from build123d import *
from OCP.BRepFilletAPI import BRepFilletAPI_MakeChamfer

# Parameters (mm, degrees)
SKETCH1_W                       = 16.6
SKETCH1_H                       = 11.5
BOSS_EXTRUDE1_DEPTH             = 10
SKETCH2_W                       = 21
SKETCH2_H                       = 14.8
BOSS_EXTRUDE2_DEPTH             = 1.5
SKETCH3_W                       = 0.5
SKETCH3_H                       = 5
BOSS_EXTRUDE3_DEPTH             = 8
SKETCH4_W                       = 0.5
SKETCH4_H                       = 0.4
CUT_EXTRUDE1_DEPTH              = 22.623424798
BOSS_EXTRUDE4_REACH             = 19.241
SKETCH5_W                       = 0.75
SKETCH5_H                       = 2.5
BOSS_EXTRUDE4_DIRECTION_2_REACH = 19.241
BOSS_EXTRUDE5_DEPTH             = 2.8
CHAMFER1_SIZE                   = 1.8
CHAMFER1_SIZE_2                 = 1.039230485
BOSS_EXTRUDE6_DEPTH             = 4.65
SKETCH8_W                       = 1.1
SKETCH8_H                       = 0.45
BOSS_EXTRUDE7_DEPTH             = 1.9
CHAMFER2_SIZE                   = 0.5
CHAMFER2_SIZE2                  = 0.288675135


with BuildPart() as part:
    # Sketch1 → Boss-Extrude1 (new body)
    with BuildSketch(Plane.XY):
        Rectangle(SKETCH1_W, SKETCH1_H)
    extrude(amount=BOSS_EXTRUDE1_DEPTH)

    # Sketch2 → Boss-Extrude2 (add)
    with BuildSketch(Plane.XY.offset(10)):
        Rectangle(SKETCH2_W, SKETCH2_H)
    extrude(amount=BOSS_EXTRUDE2_DEPTH)

    # Sketch3 → Boss-Extrude3 (add)
    with BuildSketch(Plane(origin=(0, 0, 0), x_dir=(-1, 0, 0), z_dir=(0, 0, -1))):
        Rectangle(SKETCH3_W, SKETCH3_H)
        with Locations((-6, 0)):
            Rectangle(SKETCH3_W, SKETCH3_H)
    extrude(amount=BOSS_EXTRUDE3_DEPTH)

    # Sketch4 → Cut-Extrude1 (cut, through all)
    with BuildSketch(Plane(origin=(6.25, 0, 0), x_dir=(0, 0, -1), z_dir=(1, 0, 0))):
        Polygon((6.5, 2.5), (8, 1.449688693), (8, 2.5), align=None)
        Polygon((8, -2.5), (8, -1.449688693), (6.5, -2.5), align=None)
        with Locations((2.25, -2.3)):
            Rectangle(SKETCH4_W, SKETCH4_H)
        with BuildLine():
            ThreePointArc((0, -0.75), (0.530330086, -0.530330086), (0.75, 0))
            Line((0.75, 0), (0, 0))
            Line((0, 0), (0, -0.75))
        make_face()
        with BuildLine():
            Line((0, 0), (0.75, 0))
            ThreePointArc((0.75, 0), (0.530330086, 0.530330086), (0, 0.75))
            Line((0, 0.75), (0, 0))
        make_face()
        with Locations((2.25, 2.3)):
            Rectangle(SKETCH4_W, SKETCH4_H)
        with BuildLine():
            Line((4.25, 0), (6.3, 0))
            Line((6.3, 0), (5.432692308, 0.612598863))
            ThreePointArc((5.432692308, 0.612598863), (4.655050171, 0.665965176), (4.25, 0))
        make_face()
        with BuildLine():
            Line((5.432692308, -0.612598863), (6.3, 0))
            Line((6.3, 0), (4.25, 0))
            ThreePointArc((4.25, 0), (4.655050171, -0.665965176), (5.432692308, -0.612598863))
        make_face()
    extrude(amount=-CUT_EXTRUDE1_DEPTH, mode=Mode.SUBTRACT)

    # Boss-Extrude4: up to this face of the body (flat: up to its plane)
    boss_extrude4_end = Plane(part.part.faces().sort_by_distance((0, 5.75, 5))[0])
    # Sketch5 → Boss-Extrude4 (add, up to the picked face)
    with BuildSketch(Plane(origin=(0, 0, 0), x_dir=(1, 0, 0), z_dir=(0, 1, 0)), mode=Mode.PRIVATE) as boss_extrude4_sk1:
        with Locations((-8.675, -1.25)):
            Rectangle(SKETCH5_W, SKETCH5_H)
    boss_extrude4_tool1 = split(extrude(boss_extrude4_sk1.sketch, amount=BOSS_EXTRUDE4_REACH, mode=Mode.PRIVATE), bisect_by=boss_extrude4_end, keep=Keep.BOTH, mode=Mode.PRIVATE)
    boss_extrude4 = boss_extrude4_tool1.solids().sort_by(Axis((-8.675, 0, 1.25), (0, 1, 0)))[0]
    add(boss_extrude4)

    # Boss-Extrude4 direction 2: up to this face of the body (flat: up to its plane)
    boss_extrude4_direction_2_end = Plane(part.part.faces().sort_by_distance((0, -5.75, 5))[0])
    # Sketch5 → Boss-Extrude4 direction 2 (add, up to the picked face)
    with BuildSketch(Plane(origin=(0, 0, 0), x_dir=(1, 0, 0), z_dir=(0, 1, 0)), mode=Mode.PRIVATE) as boss_extrude4_direction_2_sk1:
        with Locations((-8.675, -1.25)):
            Rectangle(SKETCH5_W, SKETCH5_H)
    boss_extrude4_direction_2_tool1 = split(extrude(boss_extrude4_direction_2_sk1.sketch, amount=-BOSS_EXTRUDE4_DIRECTION_2_REACH, mode=Mode.PRIVATE), bisect_by=boss_extrude4_direction_2_end, keep=Keep.BOTH, mode=Mode.PRIVATE)
    boss_extrude4_direction_2 = boss_extrude4_direction_2_tool1.solids().sort_by(Axis((-8.675, 0, 1.25), (0, -1, 0)))[0]
    add(boss_extrude4_direction_2)

    # Mirror1: Boss-Extrude4, Boss-Extrude4 direction 2 across plane
    add(boss_extrude4.mirror(Plane(origin=(0, 0, 0), x_dir=(0, 0, 1), z_dir=(1, 0, 0))))
    add(boss_extrude4_direction_2.mirror(Plane(origin=(0, 0, 0), x_dir=(0, 0, 1), z_dir=(1, 0, 0))))

    # Sketch6 → Boss-Extrude5 (add, symmetric)
    with BuildSketch(Plane(origin=(0, 0, 0), x_dir=(1, 0, 0), z_dir=(0, 1, 0))):
        with BuildLine():
            Line((-8.3, -2.5), (-9.05, -2.5))
            Line((-9.05, -2.5), (-10.056775734, -6.054415838))
            ThreePointArc((-10.056775734, -6.054415838), (-10.16130334, -6.692525863), (-10.056775734, -7.330635888))
            Line((-10.056775734, -7.330635888), (-9.03, -10))
            Line((-9.03, -10), (-8.3, -10))
            Line((-8.3, -10), (-8.3, -9.83))
            Line((-8.3, -9.83), (-9.324133061, -7.167955242))
            ThreePointArc((-9.324133061, -7.167955242), (-9.430562185, -6.777402526), (-9.37345004, -6.376657238))
            Line((-9.37345004, -6.376657238), (-8.3, -2.62))
            Line((-8.3, -2.62), (-8.3, -2.5))
        make_face()
    boss_extrude5 = extrude(amount=BOSS_EXTRUDE5_DEPTH, both=True)

    # Mirror2: Boss-Extrude5 across plane
    add(boss_extrude5.mirror(Plane(origin=(0, 0, 0), x_dir=(0, 0, 1), z_dir=(1, 0, 0))))

    # Chamfer1
    # the kernel refuses this chamfer: 1.8, 1.039230485 mm, written as the material it takes off along each edge
    with BuildSketch(Plane(origin=(-15.156754358, 7.4, 11.5), x_dir=(0, 0.019326765612700948, -0.9998132206222079), z_dir=(1, 0, 0))) as chamfer1_piece_1:
        Polygon((CHAMFER1_SIZE * 0.999813220622, -CHAMFER1_SIZE * 0.0193267656127), (-CHAMFER1_SIZE_2 * 0.0193267656042, -CHAMFER1_SIZE_2 * 0.999813220181), (0, 0), align=None)
    extrude(amount=30.313508717, mode=Mode.SUBTRACT)
    with BuildSketch(Plane(origin=(-10.5, -12.056754358, 11.5), x_dir=(-0.019326765612700473, 0, -0.9998132206222079), z_dir=(0, 1, 0)), Plane(origin=(10.5, 12.056754358, 11.5), x_dir=(0.019326765612700473, 0, -0.9998132206222079), z_dir=(0, -1, 0))) as chamfer1_piece_2:
        Polygon((CHAMFER1_SIZE * 0.999813220622, -CHAMFER1_SIZE * 0.0193267656127), (-CHAMFER1_SIZE_2 * 0.0193267656042, -CHAMFER1_SIZE_2 * 0.999813220181), (0, 0), align=None)
    extrude(amount=24.113508717, mode=Mode.SUBTRACT)
    with BuildSketch(Plane(origin=(15.156754358, -7.4, 11.5), x_dir=(0, 0.9983227437537925, 0.05789386240267112), z_dir=(-1, 0, 0))) as chamfer1_piece_3:
        Polygon((CHAMFER1_SIZE_2 * 0.998322743313, CHAMFER1_SIZE_2 * 0.0578938623771), (-CHAMFER1_SIZE * 0.0578938624027, CHAMFER1_SIZE * 0.998322743754), (0, 0), align=None)
    extrude(amount=30.313508717, mode=Mode.SUBTRACT)

    # Sketch7 → Boss-Extrude6 (add, symmetric)
    with BuildSketch(Plane(origin=(0, 0, 0), x_dir=(1, 0, 0), z_dir=(0, 1, 0))):
        with BuildLine():
            Line((-7.960769515, -11.5), (7.960769515, -11.5))
            ThreePointArc((7.960769515, -11.5), (1.177888648, -13.404715365), (-4.995235012, -16.8))
            Line((-4.995235012, -16.8), (-7.960769515, -11.5))
        make_face()
    extrude(amount=BOSS_EXTRUDE6_DEPTH, both=True)

    # Sketch8 → Boss-Extrude7 (add)
    with BuildSketch(Plane(origin=(0, 0, 10), x_dir=(-1, 0, 0), z_dir=(0, 0, -1))):
        with Locations((-2.48, 5.975)):
            Rectangle(SKETCH8_W, SKETCH8_H)
        with Locations((-2.48, -5.975)):
            Rectangle(SKETCH8_W, SKETCH8_H)
        with Locations((-7.43, 5.975)):
            Rectangle(SKETCH8_W, SKETCH8_H)
        with Locations((-7.43, -5.975)):
            Rectangle(SKETCH8_W, SKETCH8_H)
        with Locations((2.48, -5.975)):
            Rectangle(SKETCH8_W, SKETCH8_H)
        with Locations((7.43, -5.975)):
            Rectangle(SKETCH8_W, SKETCH8_H)
        with Locations((2.48, 5.975)):
            Rectangle(SKETCH8_W, SKETCH8_H)
        with Locations((7.43, 5.975)):
            Rectangle(SKETCH8_W, SKETCH8_H)
    extrude(amount=BOSS_EXTRUDE7_DEPTH)

    # Chamfer2: one chamfer whose edges measure the first distance from different faces: ONE call of the kernel's chamfer builder (chamfer() names one face for all edges)
    chamfer2_edges_1 = [part.edges().sort_by_distance(p)[0] for p in [
        (2.48, 6.2, 8.1),
    ]]
    chamfer2_side_1 = [part.faces().sort_by_distance(p)[0] for p in [
        (2.48, 6.2, 9.05),
    ]]
    chamfer2_edges_2 = [part.edges().sort_by_distance(p)[0] for p in [
        (7.43, 6.2, 8.1),
    ]]
    chamfer2_side_2 = [part.faces().sort_by_distance(p)[0] for p in [
        (7.43, 6.2, 9.05),
    ]]
    chamfer2_edges_3 = [part.edges().sort_by_distance(p)[0] for p in [
        (2.48, -6.2, 8.1),
    ]]
    chamfer2_side_3 = [part.faces().sort_by_distance(p)[0] for p in [
        (2.48, -6.2, 9.05),
    ]]
    chamfer2_edges_4 = [part.edges().sort_by_distance(p)[0] for p in [
        (7.43, -6.2, 8.1),
    ]]
    chamfer2_side_4 = [part.faces().sort_by_distance(p)[0] for p in [
        (7.43, -6.2, 9.05),
    ]]
    chamfer2_edges_5 = [part.edges().sort_by_distance(p)[0] for p in [
        (-2.48, -6.2, 8.1),
    ]]
    chamfer2_side_5 = [part.faces().sort_by_distance(p)[0] for p in [
        (-2.48, -6.2, 9.05),
    ]]
    chamfer2_edges_6 = [part.edges().sort_by_distance(p)[0] for p in [
        (-7.43, -6.2, 8.1),
    ]]
    chamfer2_side_6 = [part.faces().sort_by_distance(p)[0] for p in [
        (-7.43, -6.2, 9.05),
    ]]
    chamfer2_edges_7 = [part.edges().sort_by_distance(p)[0] for p in [
        (-2.48, 6.2, 8.1),
    ]]
    chamfer2_side_7 = [part.faces().sort_by_distance(p)[0] for p in [
        (-2.48, 6.2, 9.05),
    ]]
    chamfer2_edges_8 = [part.edges().sort_by_distance(p)[0] for p in [
        (-7.43, 6.2, 8.1),
    ]]
    chamfer2_side_8 = [part.faces().sort_by_distance(p)[0] for p in [
        (-7.43, 6.2, 9.05),
    ]]
    chamfer2 = BRepFilletAPI_MakeChamfer(part.part.solid().wrapped)
    for e in chamfer2_edges_1:
        chamfer2.Add(CHAMFER2_SIZE, CHAMFER2_SIZE2, e.wrapped, chamfer2_side_1[0].wrapped)  # the first distance lies on this face
    for e in chamfer2_edges_2:
        chamfer2.Add(CHAMFER2_SIZE, CHAMFER2_SIZE2, e.wrapped, chamfer2_side_2[0].wrapped)  # the first distance lies on this face
    for e in chamfer2_edges_3:
        chamfer2.Add(CHAMFER2_SIZE, CHAMFER2_SIZE2, e.wrapped, chamfer2_side_3[0].wrapped)  # the first distance lies on this face
    for e in chamfer2_edges_4:
        chamfer2.Add(CHAMFER2_SIZE, CHAMFER2_SIZE2, e.wrapped, chamfer2_side_4[0].wrapped)  # the first distance lies on this face
    for e in chamfer2_edges_5:
        chamfer2.Add(CHAMFER2_SIZE, CHAMFER2_SIZE2, e.wrapped, chamfer2_side_5[0].wrapped)  # the first distance lies on this face
    for e in chamfer2_edges_6:
        chamfer2.Add(CHAMFER2_SIZE, CHAMFER2_SIZE2, e.wrapped, chamfer2_side_6[0].wrapped)  # the first distance lies on this face
    for e in chamfer2_edges_7:
        chamfer2.Add(CHAMFER2_SIZE, CHAMFER2_SIZE2, e.wrapped, chamfer2_side_7[0].wrapped)  # the first distance lies on this face
    for e in chamfer2_edges_8:
        chamfer2.Add(CHAMFER2_SIZE, CHAMFER2_SIZE2, e.wrapped, chamfer2_side_8[0].wrapped)  # the first distance lies on this face
    add(Compound.cast(chamfer2.Shape()), mode=Mode.REPLACE)


solid = part.part
The listing builds one solid part. Answer for the finished solid, in the listing's coordinates (mm). A direction names the side the tool comes from. Coordinates: 2 decimals unless noted, no trailing zeros. Loops run counter-clockwise (first coordinate to the right, second up) from the corner with the lowest first, then second, coordinate; pieces in that order, holes last. Notation, with made-up numbers: (60.5, 3) -> (97.5, 3) arc R22 ccw to (97.5, 28) -> close; hole circle Ø11 at (-18, -34). An arc over 180 degrees is marked (long way). Answer in a Markdown table with one row per item. Add a question column.
1. The part is cut by section B-B, the plane x = -1. Write down the section's boundary in (y, z).
2. Flat-ended cylindrical pins translate along their axes: P1, Ø0.6, axis at x = 2.5, z = 9, coming from the -Y side; P2, Ø4, axis at x = 6.5, z = 1, coming from the +Y side; P3, Ø5, axis at x = 8, z = -3.5, coming from the +Y side. Find the tip coordinate at first contact, or state that the pin passes through.
3. The part is cut by section A-A, the plane y = -4. Write down the section's boundary in (x, z), then the cut area to 3 significant figures.
4. The part is cut by section C-C, the plane y = 1.75. Count the separate pieces of the cut face and the enclosed holes in it, then the cut area to 3 significant figures.
5. Consider line 1 (Z direction, x = -8.75, y = -4.5); line 2 (X direction, y = -1.75, z = -1); line 3 (Z direction, x = -8, y = -3.75). Determine where each line is inside the solid, lowest interval first. Write a range as [from, to].
6. For faces 1 (the flat face through (-9.5, -2.8, 6.2)), 2 (the flat face through (-9.55, 0.04, 8.65)), 3 (the flat face through (9.05, 0, 1)), 4 (the flat face through (-2.5, 6.2, 9.3)), 5 (the flat face through (7.4, -6.2, 9.3)), determine the directions among +Z, -Z, +X, -X, +Y, -Y from which every point of the face is accessible in a straight line to the end or side of a thin tool.
7. Determine the mould class of faces 6 (the flat face through (-8.844, 0.039, 4.525)), 7 (the flat face through (0, 1.98, -7.24)), 8 (the cylindrical face through (1.269, 0.065, 13.367)) for opening direction X: +X half, -X half, draft (parallel to the pull), parting line (faces both ways), or undercut.
Answer below:
| question | item | result |
|---|---|---|
| 1 | outline | (-7.23, 10) -> (-5.75, 10) -> (-5.75, 0) -> (5.75, 0) -> (5.75, 10) -> (7.23, 10) -> (6.36, 11.5) -> (4.65, 11.5) -> (4.65, 14.4) -> (-4.65, 14.4) -> (-4.65, 11.5) -> (-6.36, 11.5) -> close |
| 2 | P1 | y = -6.2 |
| 2 | P2 | y = 5.75 |
| 2 | P3 | y = 2.5 |
| 3 | outline | (-10.33, 10) -> (-8.3, 10) -> (-8.3, 2.5) -> (-9.05, 2.5) -> (-9.05, 0) -> (9.05, 0) -> (9.05, 2.5) -> (8.3, 2.5) -> (8.3, 10) -> (10.33, 10) -> (9.46, 11.5) -> (7.96, 11.5) arc R30.82 cw to (-5, 16.8) -> (-7.96, 11.5) -> (-9.46, 11.5) -> close |
| 3 | area | 234 mm2 |
| 4 | separate pieces | 1 |
| 4 | enclosed holes | 2 |
| 4 | area | 253 mm2 |
| 5 | line 1 | [0, 2.5], [10, 11.5] |
| 5 | line 2 | [-0.25, 0.25], [5.75, 6.25] |
| 5 | line 3 | [0, 11.5] |
| 6 | face 1 | -X, -Y |
| 6 | face 2 | -X, +Y, -Y |
| 6 | face 3 | -Z, +X, +Y, -Y |
| 6 | face 4 | -Z, +X, -X, +Y |
| 6 | face 5 | -Z, +X, -X, -Y |
| 7 | face 6 | undercut |
| 7 | face 7 | draft |
| 7 | face 8 | +X half |
